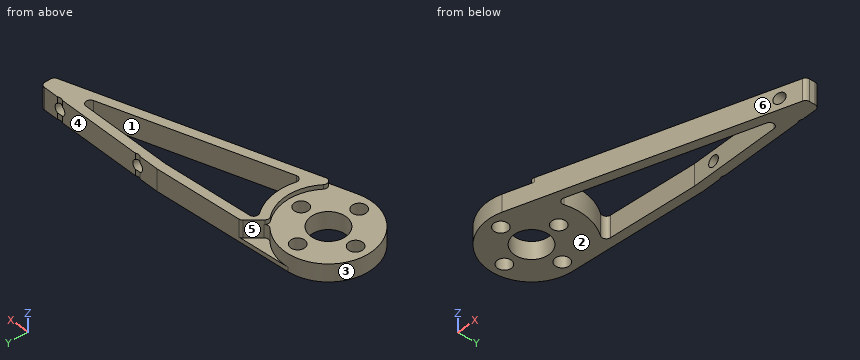
Autodesk Inventor part; units mm, degrees
ref_plane "YZ Plane" through (0, 0, 0) normal (1, 0, 0) x (0, 1, 0)
ref_plane "XZ Plane" through (0, 0, 0) normal (0, 1, 0) x (-1, 0, 0)
ref_plane "XY Plane" through (0, 0, 0) normal (0, 0, 1) x (1, 0, 0)
sketch "スケッチ1" plane through (0, 0, 0) normal (0, 0, 1) x (1, 0, 0)
  circle A0 centre (0, 0) radius 10
  line L0 (30, 12.5) -> (60, 12.5)
  line L1 (60, 12.5) -> (60, 9.5)
  line L2 (60, 9.5) -> (30, 9.5)
  line L3 (30, 9.5) -> (30, 12.5)
  line L4 (30, 12.5) -> (-0.819325, 9.966379)
  line L5 (3.168424, -9.484782) -> (60, 9.5)
  dimension "d0" = 20
  dimension "d1" = 30
  dimension "d2" = 3
  dimension "d3" = 12.5
  dimension "d4" = 60
extrude "プレート1" add sketch "スケッチ1" along normal blind 5
sketch "スケッチ2" plane through (0, 0, 5) normal (0, 0, 1) x (1, 0, 0)
  arc A0 (-0.819325, 9.966379) -> (3.168424, -9.484782) centre (0, 0) ccw
  line L0 (30, 12.5) -> (-0.819325, 9.966379)
  circle A1 centre (0, 0) radius 10
  point P0 (3.168424, -9.484782)
extrude "押し出し1" cut sketch "スケッチ2" against normal blind 1
sketch "スケッチ3" plane through (0, 0, 4) normal (0, 0, 1) x (1, 0, 0)
  circle A0 centre (0, 0) radius 7 construction
  line L0 (0, -7) -> (7, 0) construction
  line L1 (7, 0) -> (0, 7) construction
  line L2 (0, 7) -> (-7, 0) construction
  line L3 (-7, 0) -> (0, -7) construction
  line L4 (0, -7) -> (0, 7) construction
  line L5 (7, 0) -> (-7, 0) construction
  dimension "d8" = 14
hole "穴1" at (0, 7, 4) at (7, 0, 4) at (0, -7, 4) at (-7, 0, 4) direction (0, 0, -1) diameter 3.2 end through all
sketch "スケッチ4" plane through (0, 0, 4) normal (0, 0, 1) x (1, 0, 0)
  circle A0 centre (0, 0) radius 4
  dimension "d16" = 8
extrude "押し出し2" cut sketch "スケッチ4" against normal through all
sketch "スケッチ6" plane through (0, 0, 5) normal (0, 0, 1) x (1, 0, 0)
  line L0 (60, 9.5) -> (3.168424, -9.484782)
  line L1 (60, 12.5) -> (60, 9.5)
  line L2 (30, 12.5) -> (60, 12.5)
  line L3 (-0.819325, 9.966379) -> (30, 12.5)
  arc A0 (3.168424, -9.484782) -> (-0.819325, 9.966379) centre (0, 0) ccw
  line L4 (30.08207, 10.5) -> (56.681246, 10.5)
  line L5 (56.681246, 10.5) -> (11.018186, -4.753901)
  arc A1 (11.018186, -4.753901) -> (8.258741, 8.705929) centre (0, 0) ccw
  line L6 (8.258741, 8.705929) -> (30.08207, 10.5)
  dimension "d28" = 2
extrude "押し出し4" cut sketch "スケッチ6" against normal through all contours L4 L5 A1 L6
sketch "スケッチ5" plane through (0, 0, 5) normal (0, 0, 1) x (1, 0, 0)
  line L0 (30, 12.5) -> (60, 12.5)
  circle A0 centre (35, 13.35) radius 1.05
  circle A1 centre (55, 13.35) radius 1.05
  line L1 (60, 12.5) -> (60, 9.5)
  point P0 (0, 0)
  dimension "d20" = 2.1
  dimension "d21" = 2.1
  dimension "d22" = 5
  dimension "d23" = 5
  dimension "d24" = 0.85
  dimension "d25" = 0.85
extrude "押し出し3" cut sketch "スケッチ5" against normal through all
fillet "フィレット2" radius 1 4 edges at (11.0182, -4.7539, 2.5) (8.2587, 8.7059, 2.5) (56.6812, 10.5, 2.5) (30.0821, 10.5, 2.5)
sketch "スケッチ7" plane through (35.616441, 12.5, 0) normal (0, 1, 0) x (1, 0, 0)
  line L0 (18.767117, -5) -> (18.767117, 0)
  line L1 (20, -5) -> (18.767117, -5)
  line L2 (20, 0) -> (20, -5)
  line L3 (18.767117, 0) -> (20, 0)
  line L4 (-1.232883, -5) -> (-1.232883, 0)
  line L5 (0, -5) -> (-1.232883, -5)
  line L6 (0, 0) -> (0, -5)
  line L7 (-1.232883, 0) -> (0, 0)
  point P0 (-35.616441, 0)
  point P1 (-0.616441, -2.5)
  point P2 (19.383559, -2.5)
  point P3 (19.383559, -5)
  point P4 (-0.616441, -5)
  point P5 (-1.232883, -2.5)
  point P6 (18.767117, -2.5)
hole "穴2" at (35, 12.5, 2.5) at (55, 12.5, 2.5) direction (0, -1, 0) diameter 2.5 depth 8 tip angle 118
fillet "フィレット3" radius 1 3 edges at (60, 9.5, 2.5) (60, 12.5, 2.5) (30, 12.5, 2.5)
sketch "スケッチ8" plane through (0, 0, 5) normal (0, 0, 1) x (1, 0, 0)
  arc A0 (3.168424, -9.484782) -> (-0.819325, 9.966379) centre (0, 0) ccw
  line L0 (-0.819325, 9.966379) -> (29.959103, 12.496638)
  line L1 (10.269293, 10.877961) -> (7.054657, 7.08744)
  arc A1 (10.262161, 8.870628) -> (9.548394, 7.268299) centre (10.344094, 7.87399) ccw
  dimension "d40" = 2
  dimension "d41" = 45
extrude "押し出し5" cut sketch "スケッチ8" against normal blind 4
fillet "フィレット4" radius 1 4 edges at (7.0547, 7.0874, 2.5) (7.0547, 7.0874, 4.5) (10.2693, 10.878, 3) (3.1684, -9.4848, 4.5)
equation "\"d14\" = Thickness"
equation "\"d23\" = d22"
equation "\"d25\" = d24"
equation "\"d5\" = Thickness"
equation "\"BendRadius\" = Thickness"
equation "\"BendReliefWidth\" = Thickness"
equation "\"BendReliefDepth\" = 0.5 * Thickness"
equation "\"TransitionRadius\" = BendRadius"
equation "\"JacobiRadiusSize\" = BendRadius"
equation "\"GapSize\" = Thickness"
properties part number "T5.0_club-face"
Could you check a few things on this model? Use its own coordinates, in mm. Face numbers are marked on the shaded views. A direction names the side the tool comes from. Give positions to 0.01 mm unless a question says otherwise; leave off trailing zeros. Order: outer loops, then holes, each group sorted by start corner. A loop starts at its lowest first (then second) coordinate and runs counter-clockwise, first axis right, second up.
1. Will these pins go through, and if not, where does the flat tip stop? P1, Ø5, axis at x = 0, y = -7, coming from the +Z side; P2, Ø1.5, axis at x = 35, z = 2.5, coming from the +Y side; P3, Ø3, axis at x = 0, y = 7, coming from the +Z side; P4, Ø3, axis at x = 19.5, z = 2.5, coming from the -Y side.
2. For the marked faces 1, 2 and 3, which set-ups out of +Z, -Z, +X, -X, +Y, -Y let a thin tool reach every point of the face, with its end or its side?
3. Suppose I cut it at B-B (y = 0). List the corners of the cut face in (x, z) for me.
4. Suppose I cut it at A-A (z = 2.5). Give the number of separate pieces and of enclosed holes in the cut face, plus the area to 3 significant figures.
5. I need wall thicknesses on L1, parallel to Y at x = 0, z = 1.6; L2, parallel to Y at x = 1, z = 3.1; L3, parallel to Y at x = 26.5, z = 0.8. Which ranges of each line are inside material? Lowest first, please.
6. Suppose I cut it at D-D (x = 35). List the corners of the cut face in (y, z) for me.
7. We'd pull the mould along X, two halves only. Please class the marked faces 4, 5 and 6: pulls with the +X half, pulls with the -X half, needs draft (parallel to the pull), parting line crosses it, or undercut.
Solved:
1. P1: stops at z = 4
1. P2: stops at y = 3.51
1. P3: passes through
1. P4: stops at y = -4.53
2. face 1: +Z, -Z
2. face 2: -Z, +X, -X, +Y, -Y
2. face 3: +Z
3. outline: (-10, 0) - (-8.6, 0) - (-8.6, 4) - (-10, 4) - close; (-5.4, 0) - (-4, 0) - (-4, 4) - (-5.4, 4) - close; (4, 0) - (5.4, 0) - (5.4, 4) - (4, 4) - close; (8.6, 0) - (12, 0) - (12, 5) - (10, 5) - (10, 4) - (8.6, 4) - close; (25.25, 0) - (31.56, 0) - (31.56, 5) - (25.25, 5) - close
4. separate pieces: 2
4. enclosed holes: 5
4. area: 462 mm2
5. L1: y = -10 to -8.6, -5.4 to -4, 4 to 5.4, 8.6 to 10
5. L2: y = -9.95 to -8.25, -5.75 to -3.87, 3.87 to 5.75, 8.25 to 9.95
5. L3: y = -1.69 to 0.42, 10.21 to 12.21
6. outline: (1.15, 0) - (3.26, 0) - (3.26, 5) - (1.15, 5) - close; (10.5, 0) - (12.3, 0) - (12.3, 1.25) - (10.5, 1.25) - close; (10.5, 3.75) - (12.3, 3.75) - (12.3, 5) - (10.5, 5) - close
7. face 4: needs draft
7. face 5: undercut
7. face 6: pulls with the +X half
